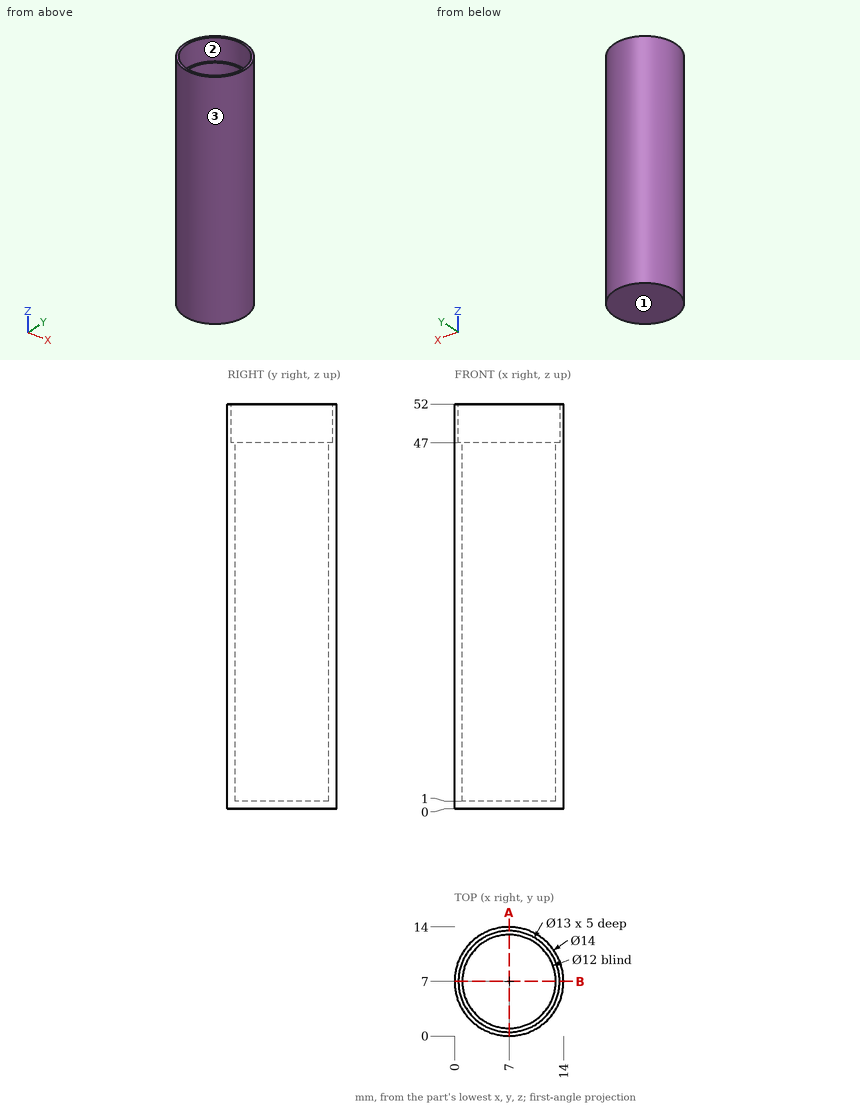
Source: three-view drawing plus pictorial views. Frame: mm from the lowest corner of the part. Give positions to 0.01 mm unless a question says otherwise; leave off trailing zeros. Order: outer loops, then holes, each group sorted by start corner. A loop starts at its lowest first (then second) coordinate and runs counter-clockwise, first axis right, second up.
1. Section A-A on x = 7. Return the cut outline in (y, z), and give its area (3 significant figures).
Derived:
outline: (0, 0) - (14, 0) - (14, 52) - (13.5, 52) - (13.5, 47) - (13, 47) - (13, 1) - (1, 1) - (1, 47) - (0.5, 47) - (0.5, 52) - (0, 52) - close
area: 111 mm2
2. Mould query, pull axis X, two halves, no side actions, for the marked faces 1, 2 and 3. Classes: released by +X, released by -X, zero draft, split by the parting line, or undercut.
Derived:
face 1: zero draft
face 2: undercut
face 3: split by the parting line
3. Material intervals for L1, parallel to Y at x = 7, z = 35; L2, parallel to Y at x = 7, z = 49.35; L3, parallel to X at y = 2, z = 17, sorted ascending.
Derived:
L1: y = 0 to 1, 13 to 14
L2: y = 0 to 0.5, 13.5 to 14
L3: x = 2.1 to 3.68, 10.32 to 11.9
4. Pin query (flat end, axial travel): pin 1 (6 mm diameter, centred on x = 12.5, z = 21.5, fed in from -Y); pin 2 (4 mm diameter, centred on x = 5.5, y = 6, fed in from +Z); pin 3 (1.5 mm diameter, centred on x = 12.5, z = 40.5, fed in from +Y). Return the tip coordinate at first contact, or that it passes through.
Derived:
pin 1: stops at y = 0.46
pin 2: stops at z = 1
pin 3: stops at y = 12.14
